Could you check a few things on this drawing? It's one solid part, dimensions in mm from its lowest x, y, z. A direction names the side the tool comes from. Round coordinates to 2 decimals unless told otherwise and drop trailing zeros. Loops run counter-clockwise (first coordinate to the right, second up) from the corner with the lowest first, then second, coordinate; pieces in that order, holes last. Notation, with made-up numbers: (-36.5, 88.5) -> (17.5, 88.5) arc R20 ccw to (17.5, 120.5) -> close; hole circle Ø4 at (59, 19). An arc over 180 degrees is marked (long way). Use one line per item in the form item = value. Start each with the question number.
Item 1: If we section it at C-C (y = 220): Write out the boundary of the cut face in (x, z), then the cut area to 3 significant figures.
Item 2: If I drill on L1, parallel to Z at x = 1.75, y = 61; L2, parallel to Z at x = 7.25, y = 202, over which ranges is the centre line in solid material (lowest first)? Write a range as [from, to].
Item 3: For the marked faces 1, 2 and 3, which set-ups out of +Z, -Z, +X, -X, +Y, -Y let a thin tool reach every point of the face, with its end or its side?
Item 4: Thinking about a two-plate mould opening in Z: for the marked faces 4, 5 and 6, which applies, released by +Z, released by -Z, zero draft, split by the parting line, or undercut?
Item 5: If we section it at D-D (z = 71.5): Write out the boundary of the cut face in (x, y) (1 decimal).
Item 6: If we section it at B-B (z = 6): Write out the boundary of the cut face in (x, y) (1 decimal).
Item 7: I'm going to push a flat-ended pin straight in: pin 1 Ø5 at (x, z) = (6.5, 42) entering from -Y. Where does the tip first touch, or does it pass through?
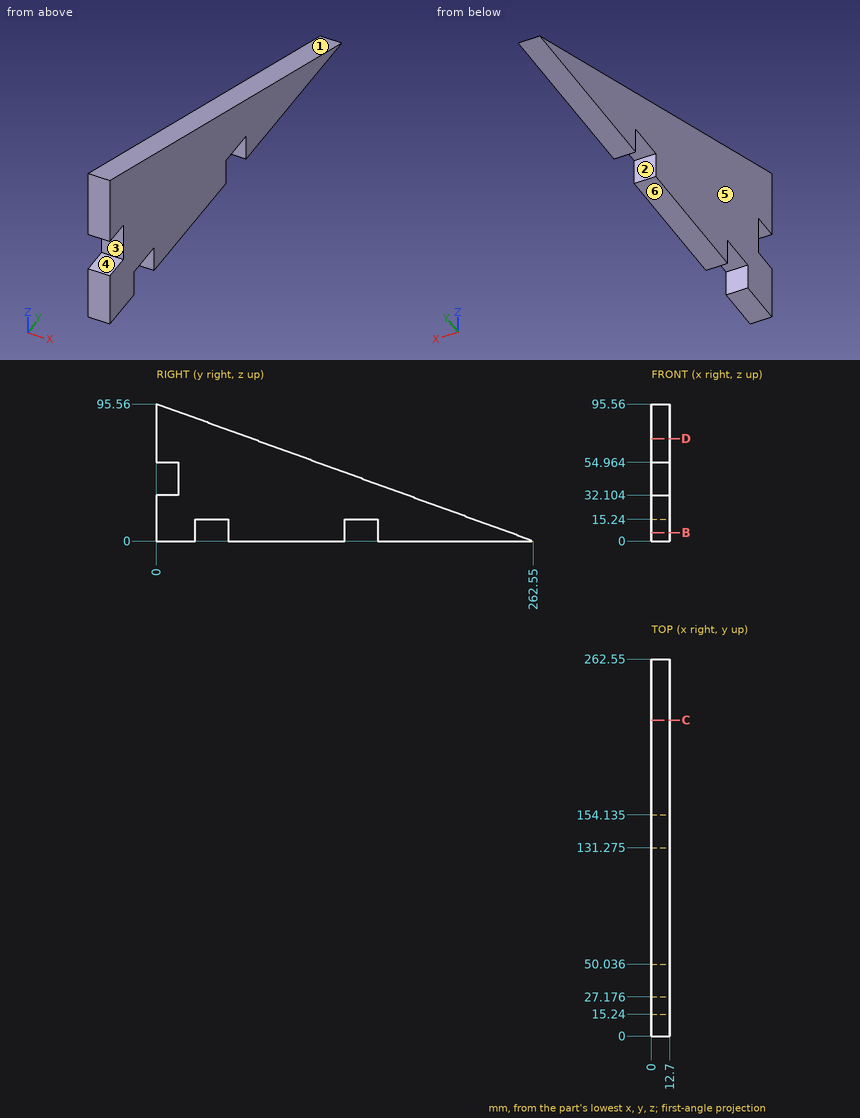
Values found:
q1.outline = (0, 0) -> (12.7, 0) -> (12.7, 15.49) -> (0, 15.49) -> close
q1.area = 197 mm2
q2.L1 = [0, 73.36]
q2.L2 = [0, 22.04]
q3.face_1 = +Z, +X, -X, +Y
q3.face_2 = -Z, +X, -X
q3.face_3 = +X, -X, -Y
q4.face_4 = undercut
q4.face_5 = zero draft
q4.face_6 = released by -Z
q5.outline = (0, 0) -> (12.7, 0) -> (12.7, 66.1) -> (0, 66.1) -> close
q6.outline = (0, 0) -> (12.7, 0) -> (12.7, 27.2) -> (0, 27.2) -> close; (0, 50) -> (12.7, 50) -> (12.7, 131.3) -> (0, 131.3) -> close; (0, 154.1) -> (12.7, 154.1) -> (12.7, 246.1) -> (0, 246.1) -> close
q7.pin_1 = 15.24
